Design review of the part built by this model. Coordinates are the model's own, in mm. A direction names the side the tool comes from. Give positions to 0.01 mm unless a question says otherwise; leave off trailing zeros. Write each loop counter-clockwise with the first axis right and the second up, starting at its lowest first coordinate (ties: lowest second). Pieces come first, ordered by that corner, then holes. Notation, with made-up numbers: M 3.25,-3.5 L 59.25,-3.5 A19 cw 59.25,3.5 Z; hole C 34.25,36.5 d1. An arc over 180 degrees is marked long. One line per item, written item: value. Start each with the question number.
```python
from build123d import *

# Parameters (mm, degrees)
SKETCH_1_W           = 210
SKETCH_1_H           = 230
EXTRUDE_1_DEPTH      = 6
SKETCH_2_W           = 9.85
SKETCH_2_H           = 208.5
EXTRUDE_3_DEPTH      = 15
SKETCH_3_R           = 2
CUT_EXTRUDE_1_DEPTH  = 10
SKETCH_17_W          = 6
SKETCH_17_H          = 230
EXTRUDE_9_DEPTH      = 66
EXTRUDE_10_DEPTH     = 6
CHAMFER_3_SIZE       = 8
SKETCH_21_R          = 2.3
CUT_EXTRUDE_9_DEPTH  = 6
SKETCH_34_R          = 2.25
CUT_EXTRUDE_14_DEPTH = 30
SKETCH_36_R          = 2.25
CUT_EXTRUDE_15_DEPTH = 30
SKETCH_51_W          = 194
SKETCH_51_H          = 230
EXTRUDE_22_DEPTH     = 4
CHAMFER_6_SIZE       = 4
CUT_EXTRUDE_START    = -5
SKETCH_54_R          = 4.75
SKETCH_54_R_2        = 2.3
CUT_EXTRUDE_21_DEPTH = 5
CUT_EXTRUDE_23_REACH = 324.062
SKETCH_60_W          = 25
SKETCH_60_H          = 30
SKETCH_61_W          = 3
SKETCH_61_H          = 3
EXTRUDE_25_DEPTH     = 230
SKETCH_63_W          = 5
SKETCH_63_H          = 8
EXTRUDE_26_DEPTH     = 3
SKETCH_65_W          = 5
SKETCH_65_H          = 8
EXTRUDE_27_DEPTH     = 3
SKETCH_64_R          = 1.15
CUT_EXTRUDE_24_DEPTH = 9
SKETCH_66_W          = 5
SKETCH_66_H          = 8
EXTRUDE_28_DEPTH     = 3
SKETCH_67_W          = 5
SKETCH_67_H          = 8
EXTRUDE_29_DEPTH     = 3
SKETCH_68_R          = 1.15
CUT_EXTRUDE_25_DEPTH = 9
SKETCH_69_W          = 10
SKETCH_69_H          = 20
EXTRUDE_30_DEPTH     = 20
SKETCH_70_W          = 10
SKETCH_70_H          = 20
EXTRUDE_31_DEPTH     = 20
SKETCH_72_R          = 2.25
CUT_EXTRUDE_26_DEPTH = 20


with BuildPart() as part:
    # 草图1 → 凸台-拉伸1 (new body)
    with BuildSketch(Plane.XY):
        with Locations((105, 115)):
            Rectangle(SKETCH_1_W, SKETCH_1_H)
    extrude(amount=EXTRUDE_1_DEPTH)

    # 草图2 → 凸台-拉伸3 (add)
    with BuildSketch(Plane(origin=(0, 0, 0), x_dir=(-1, 0, 0), z_dir=(0, 0, -1))):
        with Locations((-197, 115)):
            Rectangle(SKETCH_2_W, SKETCH_2_H)
        with Locations((-10, 115)):
            Rectangle(SKETCH_2_W, SKETCH_2_H)
    extrude(amount=EXTRUDE_3_DEPTH)

    # 草图3 → 切除-拉伸1 (cut)
    with BuildSketch(Plane(origin=(0, 0, 0), x_dir=(-1, 0, 0), z_dir=(0, 0, -1))):
        with Locations((-169.6425573, 192.25)):
            Circle(SKETCH_3_R)
        with Locations((-150.5, 205)):
            Circle(SKETCH_3_R)
        with Locations((-150.5, 179.5)):
            Circle(SKETCH_3_R)
        with Locations(Location((-150.5, 50.5, 0), (0, 0, 180))):
            Circle(SKETCH_3_R)
        with Locations(Location((-150.5, 25, 0), (0, 0, 180))):
            Circle(SKETCH_3_R)
        with Locations(Location((-169.6425573, 37.75, 0), (0, 0, 180))):
            Circle(SKETCH_3_R)
        with Locations((-34.3574427, 192.25)):
            Circle(SKETCH_3_R)
        with Locations((-53.5, 205)):
            Circle(SKETCH_3_R)
        with Locations((-53.5, 179.5)):
            Circle(SKETCH_3_R)
        with Locations(Location((-53.5, 50.5, 0), (0, 0, 180))):
            Circle(SKETCH_3_R)
        with Locations(Location((-53.5, 25, 0), (0, 0, 180))):
            Circle(SKETCH_3_R)
        with Locations(Location((-34.3574427, 37.75, 0), (0, 0, 180))):
            Circle(SKETCH_3_R)
    extrude(amount=-CUT_EXTRUDE_1_DEPTH, mode=Mode.SUBTRACT)

    # 草图17 → 凸台-拉伸9 (add)
    with BuildSketch(Plane.XY.offset(6)):
        with Locations((3, 115)):
            Rectangle(SKETCH_17_W, SKETCH_17_H)
        with Locations((207, 115)):
            Rectangle(SKETCH_17_W, SKETCH_17_H)
    extrude(amount=EXTRUDE_9_DEPTH)

    # 草图18 → 凸台-拉伸10 (add)
    with BuildSketch(Plane.XY.offset(72)):
        Polygon((210, 230), (204, 230), (6, 230), (0, 230), (0, 0), (6, 0), (204, 0), (210, 0), align=None)
    extrude(amount=EXTRUDE_10_DEPTH)

    # 倒角3
    chamfer_3_edges = [part.edges().sort_by_distance(p)[0] for p in [
        (210, 115, 78),
        (0, 115, 78),
    ]]
    chamfer(chamfer_3_edges, length=CHAMFER_3_SIZE)

    # 草图21 → 切除-拉伸9 (cut)
    with BuildSketch(Plane.XY.offset(72)):
        with Locations((105, 130)):
            Circle(SKETCH_21_R)
        with Locations((105, 100)):
            Circle(SKETCH_21_R)
    extrude(amount=CUT_EXTRUDE_9_DEPTH, mode=Mode.SUBTRACT)

    # 草图34 → 切除-拉伸14 (cut)
    with BuildSketch(Plane(origin=(0, 0, 72), x_dir=(-1, 0, 0), z_dir=(0, 0, -1))):
        with Locations((-185.25, 115)):
            Circle(SKETCH_34_R)
        with Locations((-155.25, 115)):
            Circle(SKETCH_34_R)
    extrude(amount=-CUT_EXTRUDE_14_DEPTH, mode=Mode.SUBTRACT)

    # 草图36 → 切除-拉伸15 (cut)
    with BuildSketch(Plane(origin=(0, 0, 72), x_dir=(-1, 0, 0), z_dir=(0, 0, -1))):
        with Locations((-54.75, 115)):
            Circle(SKETCH_36_R)
        with Locations((-24.75, 115)):
            Circle(SKETCH_36_R)
    extrude(amount=-CUT_EXTRUDE_15_DEPTH, mode=Mode.SUBTRACT)

    # 草图51 → 凸台-拉伸22 (add)
    with BuildSketch(Plane.XY.offset(78)):
        with Locations((105, 115)):
            Rectangle(SKETCH_51_W, SKETCH_51_H)
    extrude(amount=EXTRUDE_22_DEPTH)

    # 倒角6
    chamfer_6_edges = [part.edges().sort_by_distance(p)[0] for p in [
        (202, 115, 82),
        (8, 115, 82),
    ]]
    chamfer(chamfer_6_edges, length=CHAMFER_6_SIZE - 0.0001)  # a hair under: the kernel refuses the full size

    # 草图54 → 切除-拉伸21 (cut)
    with BuildSketch(Plane.XY.offset(82).offset(CUT_EXTRUDE_START)):
        with Locations((54.75, 115)):
            Circle(SKETCH_54_R)
        with Locations((105, 130)):
            Circle(SKETCH_54_R_2)
        with Locations((105, 100)):
            Circle(SKETCH_54_R_2)
        with Locations((24.75, 115)):
            Circle(SKETCH_54_R)
        with Locations((155.25, 115)):
            Circle(SKETCH_54_R)
        with Locations((185.25, 115)):
            Circle(SKETCH_54_R)
    extrude(amount=CUT_EXTRUDE_21_DEPTH, mode=Mode.SUBTRACT)

    # 草图60 → 切除-拉伸23 (cut, up to next)
    with BuildSketch(Plane.ZY, mode=Mode.PRIVATE) as cut_extrude_23_sk1:
        with Locations((51.5, 115)):
            Rectangle(SKETCH_60_W, SKETCH_60_H)
    cut_extrude_23_tool1 = extrude(cut_extrude_23_sk1.sketch, amount=-CUT_EXTRUDE_23_REACH, mode=Mode.PRIVATE) & part.part
    add(cut_extrude_23_tool1.solids().sort_by_distance((0, 115, 51.5))[0], mode=Mode.SUBTRACT)

    # 草图61 → 凸台-拉伸25 (add)
    with BuildSketch(Plane.XZ):
        with Locations((7.5, 23.5)):
            Rectangle(SKETCH_61_W, SKETCH_61_H)
        with Locations((7.5, 17.5)):
            Rectangle(SKETCH_61_W, SKETCH_61_H)
        with Locations((202.5, 17.5)):
            Rectangle(SKETCH_61_W, SKETCH_61_H)
        with Locations((202.5, 23.5)):
            Rectangle(SKETCH_61_W, SKETCH_61_H)
    extrude(amount=-EXTRUDE_25_DEPTH)

    # 草图63 → 凸台-拉伸26 (add)
    with BuildSketch(Plane.XY.offset(25)):
        with Locations((11.5, 4)):
            Rectangle(SKETCH_63_W, SKETCH_63_H)
    extrude(amount=-EXTRUDE_26_DEPTH)

    # 草图65 → 凸台-拉伸27 (add)
    with BuildSketch(Plane.XY.offset(19)):
        with Locations((11.5, 4)):
            Rectangle(SKETCH_65_W, SKETCH_65_H)
    extrude(amount=-EXTRUDE_27_DEPTH)

    # 草图64 → 切除-拉伸24 (cut)
    with BuildSketch(Plane.XY.offset(25)):
        with Locations((10, 4)):
            Circle(SKETCH_64_R)
    extrude(amount=-CUT_EXTRUDE_24_DEPTH, mode=Mode.SUBTRACT)

    # 草图66 → 凸台-拉伸28 (add)
    with BuildSketch(Plane.XY.offset(25)):
        with Locations((198.5, 4)):
            Rectangle(SKETCH_66_W, SKETCH_66_H)
    extrude(amount=-EXTRUDE_28_DEPTH)

    # 草图67 → 凸台-拉伸29 (add)
    with BuildSketch(Plane.XY.offset(19)):
        with Locations((198.5, 4)):
            Rectangle(SKETCH_67_W, SKETCH_67_H)
    extrude(amount=-EXTRUDE_29_DEPTH)

    # 草图68 → 切除-拉伸25 (cut)
    with BuildSketch(Plane.XY.offset(25)):
        with Locations((200, 4)):
            Circle(SKETCH_68_R)
    extrude(amount=-CUT_EXTRUDE_25_DEPTH, mode=Mode.SUBTRACT)

    # 草图69 → 凸台-拉伸30 (add)
    with BuildSketch(Plane.XY.offset(82)):
        with Locations((17, 10)):
            Rectangle(SKETCH_69_W, SKETCH_69_H)
    extrude(amount=EXTRUDE_30_DEPTH)

    # 草图70 → 凸台-拉伸31 (add)
    with BuildSketch(Plane.XY.offset(82)):
        with Locations((193, 10)):
            Rectangle(SKETCH_70_W, SKETCH_70_H)
        with Locations((193, 220)):
            Rectangle(SKETCH_70_W, SKETCH_70_H)
        with Locations((17, 220)):
            Rectangle(SKETCH_70_W, SKETCH_70_H)
    extrude(amount=EXTRUDE_31_DEPTH)

    # 草图72 → 切除-拉伸26 (cut)
    with BuildSketch(Plane.XY.offset(102)):
        with Locations((17, 220)):
            Circle(SKETCH_72_R)
        with Locations((193, 220)):
            Circle(SKETCH_72_R)
        with Locations((193, 10)):
            Circle(SKETCH_72_R)
        with Locations((17, 10)):
            Circle(SKETCH_72_R)
    extrude(amount=-CUT_EXTRUDE_26_DEPTH, mode=Mode.SUBTRACT)


solid = part.part
```
Q1. For P1, Ø12, axis at y = 138, z = -10.5, coming from the -X side (3 decimals); P2, Ø10, axis at x = 173.5, y = 189.5, coming from the -Z side; P3, Ø4.5, axis at x = 53.5, y = 50.5, coming from the +Z side, all flat-tipped, find the tip position at first contact; note any pin that passes through.
Q2. Take a section at A-A, the plane z = 88.5. Give the boundary of the cut face in (x, y), then the cut area to 3 significant figures.
Q3. Take a section at B-B, the plane x = 40. Give the boundary of the cut face in (y, z).
Q4. The part is to be moulded in two halves that separate along X. For faces 1 (the face through (12, 220, 92)), 2 (the face through (105, 230, 73)), 3 (the face through (6, 113, 11)), say which applies: pulls with the +X half, pulls with the -X half, needs draft (parallel to the pull), parting line crosses it, or undercut.
Q5. Wall thickness on line 1 (X direction, y = 37.75, z = 3.95); line 2 (Y direction, x = 17, z = 97); line 3 (Z direction, x = 30, y = 168): over which ranges is each line inside the solid? List them lowest first. Write a range as from..to.
Q6. Machinability: for faces 4 (the face through (192.075, 114, -7)), 5 (the face through (204, 113, 11)), 6 (the face through (188, 220, 92)), 7 (the face through (184.22, 110.363, 79.465)), 8 (the face through (198, 10, 92)), which of the approach directions +Z, -Z, +X, -X, +Y, -Y give a long, thin tool a straight path to every point of the face, cutting with its end or side? Answer none if there is none.
Results list:
1. P1: stops at x = 5.075
1. P2: stops at z = 0
1. P3: stops at z = 82
2. outline: M 12,0 L 22,0 L 22,20 L 12,20 Z; M 12,210 L 22,210 L 22,230 L 12,230 Z; M 188,0 L 198,0 L 198,20 L 188,20 Z; M 188,210 L 198,210 L 198,230 L 188,230 Z; hole C 17,10 d4.5; hole C 17,220 d4.5; hole C 193,10 d4.5; hole C 193,220 d4.5
2. area: 736 mm^2
3. outline: M 0,0 L 230,0 L 230,6 L 0,6 Z; M 0,72 L 230,72 L 230,82 L 0,82 Z
4. face 1: pulls with the -X half
4. face 2: needs draft
4. face 3: undercut
5. line 1: x = 0..32.36, 36.36..167.64, 171.64..210
5. line 2: y = 0..7.75, 12.25..20, 210..217.75, 222.25..230
5. line 3: z = 0..6, 72..82
6. face 4: -Z, +Y, -Y
6. face 5: +Y, -Y
6. face 6: +Z, +Y, -Y
6. face 7: +Z
6. face 8: +Z, +X, +Y, -Y
